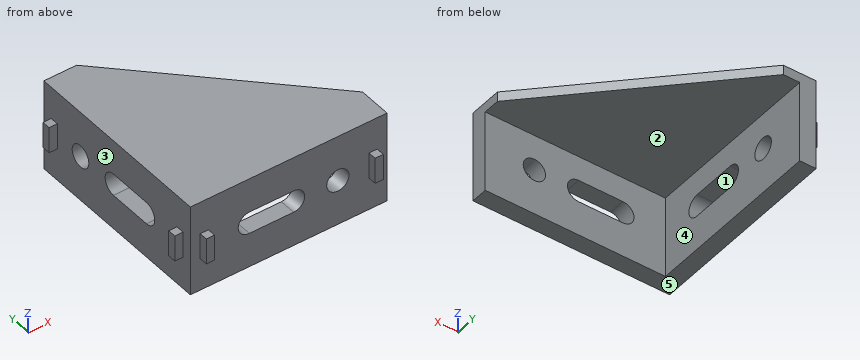
from build123d import *

# Parameters (mm, degrees)
EXTRUDE_1_DEPTH     = 14
EXTRUDE_2_DEPTH     = 3
SKETCH_3_R          = 3.4
CUT_EXTRUDE_1_DEPTH = 6
SKETCH_4_W          = 2.5
SKETCH_4_H          = 8
EXTRUDE_3_DEPTH     = 2.5


with BuildPart() as part:
    # Эскиз1 → Бобышка-Вытянуть1 (new body, symmetric)
    with BuildSketch(Plane.XY):
        Polygon((0, 60), (0, 0), (60, 0), (60, 5), (5, 5), (5, 60), align=None)
    extrude(amount=EXTRUDE_1_DEPTH, both=True)

    # Эскиз2 → Бобышка-Вытянуть2 (add)
    with BuildSketch(Plane.XY.offset(14)):
        Polygon((60, 5), (5, 5), (5, 60), (10, 60), (60, 10), align=None)
    extrude(amount=-EXTRUDE_2_DEPTH)

    # Эскиз3 → Вырез-Вытянуть1 (cut, through all)
    with BuildSketch(Plane(origin=(0, 5, 0), x_dir=(1, 0, 0), z_dir=(0, 1, 0))):
        with Locations(Location((45, 0, 0), (0, 0, 270))):  # turned: the seam where the file's is
            Circle(SKETCH_3_R)
        with BuildLine():
            Line((18, 3.4), (31.5, 3.4))
            ThreePointArc((31.5, 3.4), (34.9, 0), (31.5, -3.4))
            Line((31.5, -3.4), (18, -3.4))
            ThreePointArc((18, -3.4), (14.6, 0), (18, 3.4))
        make_face()
    cut_extrude_1 = extrude(amount=-CUT_EXTRUDE_1_DEPTH, mode=Mode.SUBTRACT)

    # Эскиз4 → Бобышка-Вытянуть3 (add)
    with BuildSketch(Plane.XZ):
        with Locations((4.25, 0)):
            Rectangle(SKETCH_4_W, SKETCH_4_H)
        with Locations((55.75, 0)):
            Rectangle(SKETCH_4_W, SKETCH_4_H)
    extrude_3 = extrude(amount=EXTRUDE_3_DEPTH)

    # Зеркальное отражение3: Вырез-Вытянуть1, Бобышка-Вытянуть3 across plane
    add(cut_extrude_1.mirror(Plane(origin=(0, 0, 0), x_dir=(0, 0, 1), z_dir=(-0.707106781, 0.707106781, 0))), mode=Mode.SUBTRACT)
    add(extrude_3.mirror(Plane(origin=(0, 0, 0), x_dir=(0, 0, 1), z_dir=(-0.707106781, 0.707106781, 0))))


solid = part.part
Check sheet for the modelled part. Datum: model origin and axes. Units: mm. Face numbers are marked on the shaded views. A direction names the side the tool comes from. Give positions to 0.01 mm unless a question says otherwise; leave off trailing zeros. Loops run counter-clockwise (first coordinate to the right, second up) from the corner with the lowest first, then second, coordinate; pieces in that order, holes last. Notation, with made-up numbers: M 50.5,58 L 63.5,58 A37 ccw 63.5,95 Z; hole C 11.25,63.25 d3. An arc over 180 degrees is marked long. Use a Markdown table: item, result. Add a question column.
Q1. Mould release check, pull along Z, two halves, no side actions. Record for the marked faces 1, 2 and 3: pulls with the +Z half, pulls with the -Z half, needs draft (parallel to the pull), parting line crosses it, or undercut.
Q2. Sectioned sample at A-A, the plane x = 45. Record the cut outline in (y, z).
Q3. Sectioned sample at D-D, the plane z = -7. Record the cut outline in (x, y), then the cut area to 3 significant figures.
Q4. Go/stop test with flat-tipped pins: pin 1 (3 mm diameter, centred on y = 7.5, z = 7, fed in from +X); pin 2 (2 mm diameter, centred on x = -1.5, z = -0.5, fed in from -Y); pin 3 (2 mm diameter, centred on x = 14.5, z = -6.5, fed in from +Y). Record where each tip stops, or that it passes through.
Q5. Sectioned sample at C-C, the plane z = 0. Give the number of separate pieces and of enclosed holes in the cut face, then the cut area to 3 significant figures.
Q6. Tool access check on the marked faces 4 and 5. Record the directions out of +Z, -Z, +X, -X, +Y, -Y that give a thin tool (end or side, any length) a straight path to the whole face; none if there is none.
Q7. Sectioned sample at B-B, the plane y = 22. Record the cut outline in (x, z), then the cut area to 3 significant figures.
Q8. Scan lines: line 1 along X through (y, z) = (2.15, 0); line 2 along Y through (x, z) = (7.5, 7.5); line 3 along Z through (x, y) = (19, 21.5). Record each from-to range of solid material in increasing order. Write a range as [from, to].
Verdict:
| question | item | result |
|---|---|---|
| 1 | face 1 | undercut |
| 1 | face 2 | pulls with the -Z half |
| 1 | face 3 | needs draft |
| 2 | outline | M 0,-14 L 5,-14 L 5,-3.4 L 0,-3.4 Z; M 0,3.4 L 5,3.4 L 5,11 L 25,11 L 25,14 L 0,14 Z |
| 3 | outline | M 0,0 L 60,0 L 60,5 L 5,5 L 5,60 L 0,60 Z |
| 3 | area | 575 mm^2 |
| 4 | pin 1 | x = 5 |
| 4 | pin 2 | y = 3 |
| 4 | pin 3 | y = 5 |
| 5 | separate pieces | 5 |
| 5 | enclosed holes | 0 |
| 5 | area | 329 mm^2 |
| 6 | face 4 | -Z, +X, +Y |
| 6 | face 5 | -Z, +X, -X, +Y, -Y |
| 7 | outline | M 0,-14 L 5,-14 L 5,-3.4 L 0,-3.4 Z; M 0,3.4 L 5,3.4 L 5,11 L 48,11 L 48,14 L 0,14 Z |
| 7 | area | 235 mm^2 |
| 8 | line 1 | [0, 14.6], [34.9, 41.6], [48.4, 60] |
| 8 | line 2 | [0, 5] |
| 8 | line 3 | [11, 14] |
